Source: CAD feature listing. Evaluate the final solid. Frame: model axes, mm. A direction names the side the tool comes from. Round coordinates to 2 decimals unless told otherwise and drop trailing zeros.
```python
from build123d import *


with BuildPart() as f1:
    # F0 (on Top) → F1 (revolve)
    with BuildSketch(Plane.XY):
        Polygon((-66.6158646345, 0), (71.9380378723, 0), (71.9380378723, 55.6167066097), (62.3581297696, 55.6167066097), (62.3581297696, 49.0526966751), (54.5522719622, 49.0526966751), (54.5522719622, 41.956461966), (46.7464216053, 41.956461966), (46.7464216053, 34.8602347076), (39.1179732978, 34.8602347076), (39.1179732978, 26.8769748509), (29.892873019, 26.8769748509), (29.892873019, 19.2485246807), (22.4418267608, 19.2485246807), (22.4418267608, 12.5071061775), (15.5230062082, 12.5071061775), (15.5230062082, 5.4108761251), (8.6041800678, 5.4108761251), (8.6041800678, 1.507949084), (-5.0560631789, 1.507949084), (-5.0560631789, 6.8301218562), (-13.9263533056, 6.8301218562), (-13.9263533056, 12.5071061775), (-23.6836709082, 12.5071061775), (-23.6836709082, 18.1840918958), (-31.4895249903, 18.1840918958), (-31.4895249903, 25.2803210169), (-37.3439155519, 25.2803210169), (-37.3439155519, 33.6183905602), (-42.843490839, 33.6183905602), (-42.843490839, 40.7146215439), (-49.2300987244, 40.7146215439), (-49.2300987244, 48.5204793513), (-55.0844892859, 48.5204793513), (-55.0844892859, 170.8428710699), (-55.0844892859, 270.9693610668), (-67.9839998484, 311.6098642349), align=None)
    revolve(axis=Axis((-67.2999322414, 155.8049321175, 0), (-0.0043904965, 0.9999903617, 0)))


solid = f1.part
```
1. Access query for faces 1 (the face through (-75.69, 48.43, -8.13)), 2 (the face through (-68.495, -0.046, 8.461)), 3 (the face through (-79.287, 21.682, -95.783)). Directions: +Z, -Z, +X, -X, +Y, -Y. A direction counts if a zero-diameter tool reaches every point of the face in a straight line with its end or side. Return the directions, or none.
2. Line query: line 1 along Z through (x, y) = (-74.5, 41); line 2 along Z through (x, y) = (-40, 17.5); line 3 along Y through (x, z) = (50.5, -55). Output: solid intervals per line, ascending.
3. First-contact query: pin 1 (12 mm diameter, centred on x = -66.5, y = 181, fed in from +Z); pin 2 (1 mm diameter, centred on x = -111.5, z = 37, fed in from -Y); pin 3 (4 mm diameter, centred on x = -141.5, z = -32.5, fed in from -Y). Flat tips, straight axial feed; report the tip coordinate or a pass-through.
Result:
1. face 1: none
1. face 2: +X, -Y
1. face 3: +Y
2. line 1: z = -138.52 to -113.28, -15.79 to 15.79, 113.28 to 138.52
2. line 2: z = -136.04 to -85.04, -33.72 to 33.72, 85.04 to 136.04
2. line 3: y = -0.05 to 55.56
3. pin 1: stops at z = 12.35
3. pin 2: stops at y = -0.46
3. pin 3: stops at y = -0.7
